Check sheet for the modelled part. Datum: model origin and axes. Units: mm. Round coordinates to 2 decimals unless told otherwise and drop trailing zeros. Write each loop counter-clockwise with the first axis right and the second up, starting at its lowest first coordinate (ties: lowest second). Pieces come first, ordered by that corner, then holes. Notation, with made-up numbers: M 62.25,62 L 115.25,62 A17 ccw 115.25,94 Z; hole C -39,32 d10. An arc over 180 degrees is marked long. Put each result on its own line as item: value.
```python
from build123d import *

# Parameters (mm, degrees)
F1_DEPTH  = 533.4
F3_DEPTH  = 19.05
F5_DEPTH  = 19.05
F7_R      = 25.4
F8_DEPTH  = 19.05
F9_R      = 25.4
F10_DEPTH = 25.4


with BuildPart() as f1:
    # F0 (on Top) → F1 (new body)
    with BuildSketch(Plane.XY):
        Polygon((-257.6280923571, 552.4852269775), (0, 0), (17.265163343, 8.0508778862), (-240.3629290141, 560.5361048637), align=None)
    extrude(amount=F1_DEPTH)

    # F2 (on face) → F3 (join)
    with BuildSketch(Plane(origin=(0, 0, 0), x_dir=(1, 0, 0), z_dir=(0, 0, -1))):
        Polygon((-225.056502435, -482.6352269775), (-207.791339092, -490.6861048637), (-186.3223313955, -444.6456692822), (-203.5874947386, -436.5947913961), align=None)
        Polygon((-171.0159048164, -366.7447913961), (-153.7507414734, -374.7956692822), (-132.281733777, -328.7552337008), (-149.54689712, -320.7043558146), align=None)
        Polygon((-116.9753071979, -250.8543558146), (-99.7101438548, -258.9052337008), (-78.2411361584, -212.8647981193), (-95.5062995015, -204.8139202332), align=None)
        Polygon((-62.9347095793, -134.9639202332), (-45.6695462363, -143.0147981193), (-24.2005385399, -96.9743625379), (-41.4657018829, -88.9234846517), align=None)
    extrude(amount=F3_DEPTH)

    # F4 (on face) → F5 (join)
    with BuildSketch(Plane.XY.offset(533.4)):
        Polygon((-207.791339092, 490.6861048637), (-225.056502435, 482.6352269775), (-203.5874947386, 436.5947913961), (-186.3223313955, 444.6456692822), align=None)
        Polygon((-171.0159048164, 366.7447913961), (-149.54689712, 320.7043558146), (-132.281733777, 328.7552337008), (-153.7507414734, 374.7956692822), align=None)
        Polygon((-78.2411361584, 212.8647981193), (-99.7101438548, 258.9052337008), (-116.9753071979, 250.8543558146), (-95.5062995015, 204.8139202332), align=None)
        Polygon((-24.2005385399, 96.9743625379), (-45.6695462363, 143.0147981193), (-62.9347095793, 134.9639202332), (-41.4657018829, 88.9234846517), align=None)
    extrude(amount=F5_DEPTH)

    # F7 (on face) → F8 (cut)
    with BuildSketch(Plane(origin=(0, 0, 0), x_dir=(0.4226182617, -0.906307787, 0), z_dir=(-0.906307787, -0.4226182617, 0))):
        with Locations((-98.1162094419, 431.8)):
            Circle(F7_R)
        with Locations((-98.1162094419, 101.6)):
            Circle(F7_R)
        with Locations((-353.8581047209, 101.6)):
            Circle(F7_R)
        with Locations((-481.7290523605, 101.6)):
            Circle(F7_R)
        with Locations((-225.9871570814, 101.6)):
            Circle(F7_R)
        with Locations((-225.9871570814, 431.8)):
            Circle(F7_R)
        with Locations((-353.8581047209, 431.8)):
            Circle(F7_R)
        with Locations((-481.7290523605, 431.8)):
            Circle(F7_R)
    extrude(amount=-F8_DEPTH, mode=Mode.SUBTRACT)

    # F9 (on face) → F10 (cut)
    with BuildSketch(Plane(origin=(17.265163343, 8.0508778862, 0), x_dir=(-0.4226182617, 0.906307787, 0), z_dir=(0.906307787, 0.4226182617, 0))):
        with Locations((481.7290523605, 266.7)):
            Circle(F9_R)
        with Locations((98.1162094419, 266.7)):
            Circle(F9_R)
    extrude(amount=-F10_DEPTH, mode=Mode.SUBTRACT)


solid = f1.part
```
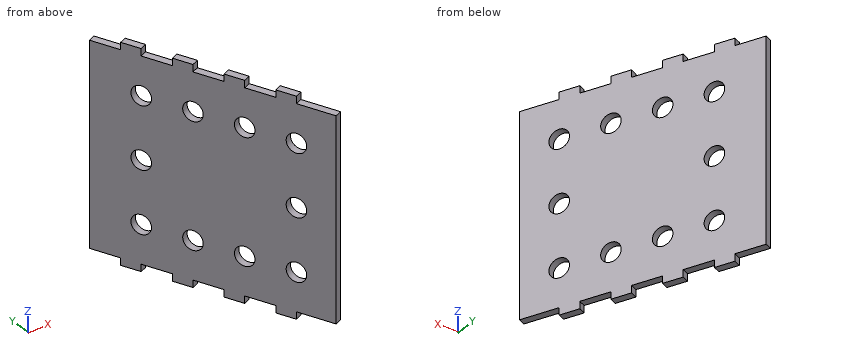
1. Depth check by flat-ended pin: pin 1 Ø8 at (y, z) = (274.5, 298.5) entering from +X; pin 2 Ø5 at (x, z) = (-37.5, 493.5) entering from +Y; pin 3 Ø1.5 at (x, z) = (-96.5, 94) entering from -Y. Enter the tip coordinate at first touch or a pass-through.
Computed values:
pin 1: stops at x = -105.12
pin 2: stops at y = 130.86
pin 3: stops at y = 230.65
2. Scan lines: probe 1 along Z at (x, y) = (-37, 114.5); probe 2 along X at (y, z) = (39.5, 38); probe 3 along X at (y, z) = (57.5, 32). Record each from-to range of solid material in increasing order.
Computed values:
probe 1: z = -19.05 to 87.75, 115.45 to 252.85, 280.55 to 417.95, 445.65 to 552.45
probe 2: x = -18.42 to 2.6
probe 3: x = -26.81 to -5.79
3. Cross-section at A-A (z = 467.5). Enter the section's corners in (x, y).
Computed values:
outline: M -257.63,552.49 L 0,0 L 17.27,8.05 L -240.36,560.54 Z
4. Cross-section at B-B (y = 395). Enter the section's corners in (x, z).
Computed values:
outline: M -184.19,0 L -163.17,0 L -163.17,533.4 L -184.19,533.4 Z
